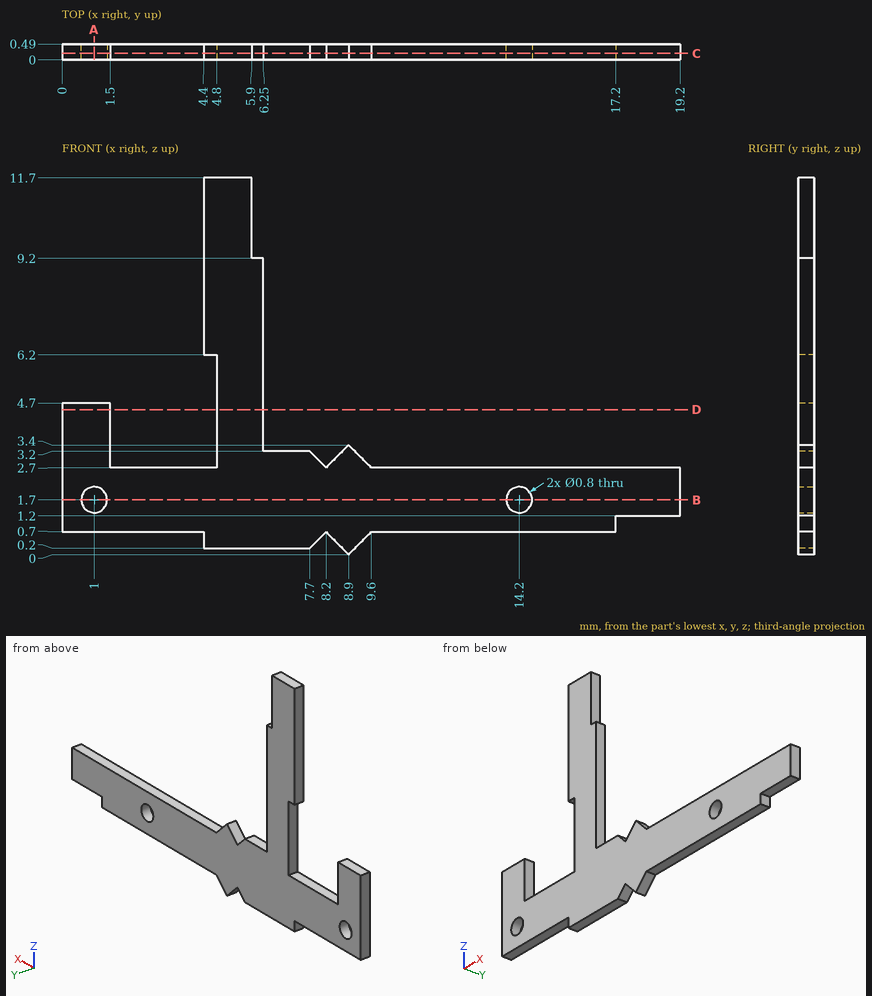
Part print with two shaded views. Sizes in mm from the minimum x, y, z corner. Coordinates: 2 decimals unless noted, no trailing zeros. Loops run counter-clockwise (first coordinate to the right, second up) from the corner with the lowest first, then second, coordinate; pieces in that order, holes last. Notation, with made-up numbers: M 40.5,70 L 78.5,70 A15 ccw 78.5,78 Z; hole C 21,43.25 d9. An arc over 180 degrees is marked long. Use CSV: the item, a comma, the result in double quotes. Start each with the question number.
1. Band-saw the part on A-A, the plane x = 1. List the corners of the cut face in (y, z), then the cut area to 3 significant figures.
2. Probe probe 1 along Z at (x, y) = (1, 0.4); probe 2 along Z at (x, y) = (4.75, 0.3); probe 3 along X at (y, z) = (0.2, 7). List the from-to ranges inside material, lowest first. Write a range as [from, to].
3. Band-saw the part on B-B, the plane z = 1.7. List the corners of the cut face in (x, y), then the cut area to 3 significant figures.
4. Band-saw the part on C-C, the plane y = 0.2. List the corners of the cut face in (x, z).
5. Band-saw the part on D-D, the plane z = 4.5. List the corners of the cut face in (x, y).
Entries:
1,outline,"M 0,0.7 L 0.49,0.7 L 0.49,1.3 L 0,1.3 Z; M 0,2.1 L 0.49,2.1 L 0.49,4.7 L 0,4.7 Z"
1,area,"1.57 mm2"
2,probe 1,"z = [0.7, 1.3], [2.1, 4.7]"
2,probe 2,"z = [0.2, 2.7], [6.2, 11.7]"
2,probe 3,"x = [4.4, 6.25]"
3,outline,"M 0,0 L 0.6,0 L 0.6,0.49 L 0,0.49 Z; M 1.4,0 L 13.8,0 L 13.8,0.49 L 1.4,0.49 Z; M 14.6,0 L 19.2,0 L 19.2,0.49 L 14.6,0.49 Z"
3,area,"8.62 mm2"
4,outline,"M 0,0.7 L 4.4,0.7 L 4.4,0.2 L 7.7,0.2 L 8.2,0.7 L 8.9,0 L 9.6,0.7 L 17.2,0.7 L 17.2,1.2 L 19.2,1.2 L 19.2,2.7 L 9.6,2.7 L 8.9,3.4 L 8.2,2.7 L 7.7,3.2 L 6.25,3.2 L 6.25,9.2 L 5.9,9.2 L 5.9,11.7 L 4.4,11.7 L 4.4,6.2 L 4.8,6.2 L 4.8,2.7 L 1.5,2.7 L 1.5,4.7 L 0,4.7 Z; hole C 1,1.7 d0.8; hole C 14.2,1.7 d0.8"
5,outline,"M 0,0 L 1.5,0 L 1.5,0.49 L 0,0.49 Z; M 4.8,0 L 6.25,0 L 6.25,0.49 L 4.8,0.49 Z"
